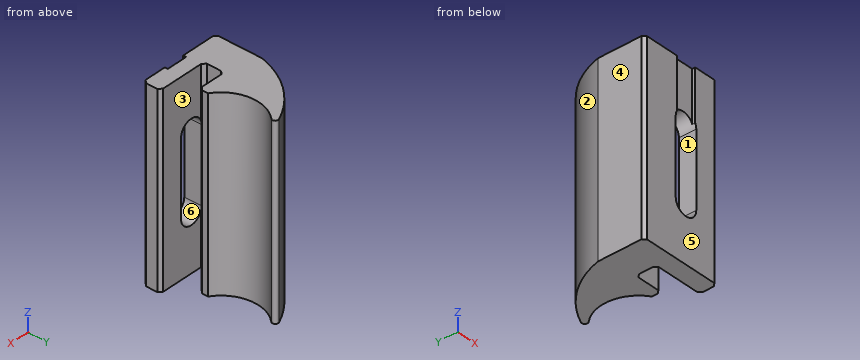
```python
from build123d import *

# Parameters (mm, degrees)
BOSS_EXTRUDE1_DEPTH     = 31.75
CHAMFER1_SIZE           = 0.508
BOSS_EXTRUDE2_DEPTH     = 2.956637053
CUT_EXTRUDE1_REACH      = 41.356
CUT_EXTRUDE2_REACH      = 48.717
CUT_EXTRUDE2_END_RADIUS = 1.9812
SKETCH7_W               = 3.556
SKETCH7_H               = 1.016


with BuildPart() as part:
    # Sketch1 → Boss-Extrude1 (new body)
    with BuildSketch(Plane.XY):
        with BuildLine():
            Line((0, 12.7), (13.97, 12.7))
            Line((13.97, 12.7), (13.97, 15.656637053))
            Line((13.97, 15.656637053), (5.588, 15.656637053))
            Line((5.588, 15.656637053), (5.588, 19.119334391))
            Line((5.588, 19.119334391), (10.414, 19.119334391))
            Line((10.414, 19.119334391), (10.414, 20.643334391))
            ThreePointArc((10.414, 20.643334391), (7.568862019, 25.230360252), (9.20630181, 30.373745063))
            ThreePointArc((9.20630181, 30.373745063), (9.344088063, 31.041104373), (8.694495233, 31.246974853))
            ThreePointArc((8.694495233, 31.246974853), (3.113774689, 26.956545429), (0, 20.643334391))
            Line((0, 20.643334391), (0, 12.7))
        make_face()
    extrude(amount=-BOSS_EXTRUDE1_DEPTH)

    # Chamfer1
    chamfer1_edges = [part.edges().sort_by_distance(p)[0] for p in [
        (0, 12.7, -15.875),
        (13.97, 12.7, -15.875),
        (13.97, 15.656637053, -15.875),
        (5.588, 15.656637053, -15.875),
        (5.588, 19.119334391, -15.875),
        (10.414, 19.119334391, -15.875),
    ]]
    chamfer(chamfer1_edges, length=CHAMFER1_SIZE)

    # Sketch4 → Boss-Extrude2 (add)
    with BuildSketch(Plane.XZ.offset(-12.7)):
        with BuildLine():
            Line((6.012029018, -22.225), (6.012029018, -9.525))
            ThreePointArc((6.012029018, -9.525), (7.993229018, -7.5438), (9.974429018, -9.525))
            Line((9.974429018, -9.525), (9.974429018, -22.225))
            ThreePointArc((9.974429018, -22.225), (7.993229018, -24.2062), (6.012029018, -22.225))
        make_face()
    extrude(amount=-BOSS_EXTRUDE2_DEPTH)

    # Sketch5 → Cut-Extrude1 (cut, up to next)
    with BuildSketch(Plane.XZ.offset(-12.7), mode=Mode.PRIVATE) as cut_extrude1_sk1:
        with BuildLine():
            Line((6.012029018, -22.225), (6.012029018, -9.525))
            ThreePointArc((6.012029018, -9.525), (7.993229018, -7.5438), (9.974429018, -9.525))
            Line((9.974429018, -9.525), (9.974429018, -22.225))
            ThreePointArc((9.974429018, -22.225), (7.993229018, -24.2062), (6.012029018, -22.225))
        make_face()
    cut_extrude1_tool1 = extrude(cut_extrude1_sk1.sketch, amount=-CUT_EXTRUDE1_REACH, mode=Mode.PRIVATE) & part.part
    add(cut_extrude1_tool1.solids().sort_by_distance((7.993229, 12.7, -15.875))[0], mode=Mode.SUBTRACT)

    # Cut-Extrude2: up to this cylinder (the profile starts outside it)
    cut_extrude2_end = Plane(origin=(7.993229018, 12.7, -9.525), z_dir=(0, -1, 0)) * Cylinder(CUT_EXTRUDE2_END_RADIUS, 102.3964, mode=Mode.PRIVATE)
    # Sketch7 → Cut-Extrude2 (cut, up to the surface)
    with BuildSketch(Plane.XY, mode=Mode.PRIVATE) as cut_extrude2_sk1:
        with Locations((7.993229018, 12.7)):
            Rectangle(SKETCH7_W, SKETCH7_H)
    cut_extrude2_tool1 = extrude(cut_extrude2_sk1.sketch, amount=-CUT_EXTRUDE2_REACH, mode=Mode.PRIVATE) - cut_extrude2_end
    add(cut_extrude2_tool1.solids().sort_by_distance((7.993229, 12.7, 0))[0], mode=Mode.SUBTRACT)


solid = part.part
```
The listing builds one solid part. Answer for the finished solid, in the listing's coordinates (mm). Face numbers are marked on the shaded views. A direction names the side the tool comes from. Give positions to 0.01 mm unless a question says otherwise; leave off trailing zeros. Write each loop counter-clockwise with the first axis right and the second up, starting at its lowest first coordinate (ties: lowest second). Pieces come first, ordered by that corner, then holes. Notation, with made-up numbers: (15.5, -28) - (65.5, -28) arc R27 ccw to (65.5, -2) - close; hole circle Ø11 at (-4, 8). An arc over 180 degrees is marked (long way). Use one line per item in the form item = value. Start each with the question number.
1) Find section D-D on y = 17. Determine the outline of the cut face in (x, z), plus the area to 3 significant figures.
2) Find section B-B on x = 8. Determine the outline of the cut face in (y, z).
3) Flat-ended cylindrical pins translate along their axes: pin 1 Ø1.2 at (y, z) = (17, -19) entering from +X; pin 2 Ø8 at (y, z) = (20, -11.5) entering from +X. Find the tip coordinate at first contact, or state that the pin passes through.
4) A tool of negligible diameter and unlimited length cuts with its end or side. For the marked faces 1, 2 and 3, from which of +Z, -Z, +X, -X, +Y, -Y can it reach the whole face along a straight path? Write none if from no direction.
5) The mould has two halves that part along X. Classify the marked faces 4, 5 and 6: pulls with the +X half, pulls with the -X half, needs draft (parallel to the pull), parting line crosses it, or undercut.
6) Find section C-C on x = 11. Determine the outline of the cut face in (y, z), plus the area to 3 significant figures.
7) Consider line 1 along Y through (x, z) = (8.75, -2); line 2 along Y through (x, z) = (13, -2.5); line 3 along Z through (x, y) = (7, 15.25). Determine where each line is inside the solid, lowest interval first. Write a range as from..to.
8) Find section A-A on z = -10. Determine the outline of the cut face in (x, y).
Geometry results:
q1.outline = (0, -31.75) - (5.59, -31.75) - (5.59, 0) - (0, 0) - close
q1.area = 177 mm2
q2.outline = (12.7, -31.75) - (15.66, -31.75) - (15.66, -24.21) - (12.7, -24.21) - close; (13.21, -7.54) - (15.66, -7.54) - (15.66, 0) - (13.21, 0) - close; (19.12, -31.75) - (23.58, -31.75) - (23.58, 0) - (19.12, 0) - close; (28.47, -31.75) - (30.91, -31.75) - (30.91, 0) - (28.47, 0) - close
q3.pin_1 = 5.59
q3.pin_2 = 10.41
q4.face_1 = -Y
q4.face_2 = +Z, -Z, -X, +Y
q4.face_3 = +Z, -Z, +X
q5.face_4 = pulls with the -X half
q5.face_5 = needs draft
q5.face_6 = undercut
q6.outline = (12.7, -31.75) - (15.66, -31.75) - (15.66, 0) - (12.7, 0) - close
q6.area = 93.9 mm2
q7.line_1 = 13.21..15.66, 19.12..22.24, 29.81..31.27
q7.line_2 = 12.7..15.66
q7.line_3 = -31.75..-23.94, -7.81..0
q8.outline = (0, 13.21) - (0.51, 12.7) - (6.01, 12.7) - (6.01, 15.74) - (5.59, 16.16) - (5.59, 18.61) - (6.1, 19.12) - (9.91, 19.12) - (10.41, 19.63) - (10.41, 20.64) arc R6.45 cw to (9.21, 30.37) arc R0.51 ccw to (8.69, 31.25) arc R15.53 ccw to (0, 20.64) - close; (9.97, 12.7) - (13.46, 12.7) - (13.97, 13.21) - (13.97, 15.15) - (13.46, 15.66) - (9.97, 15.66) - close
